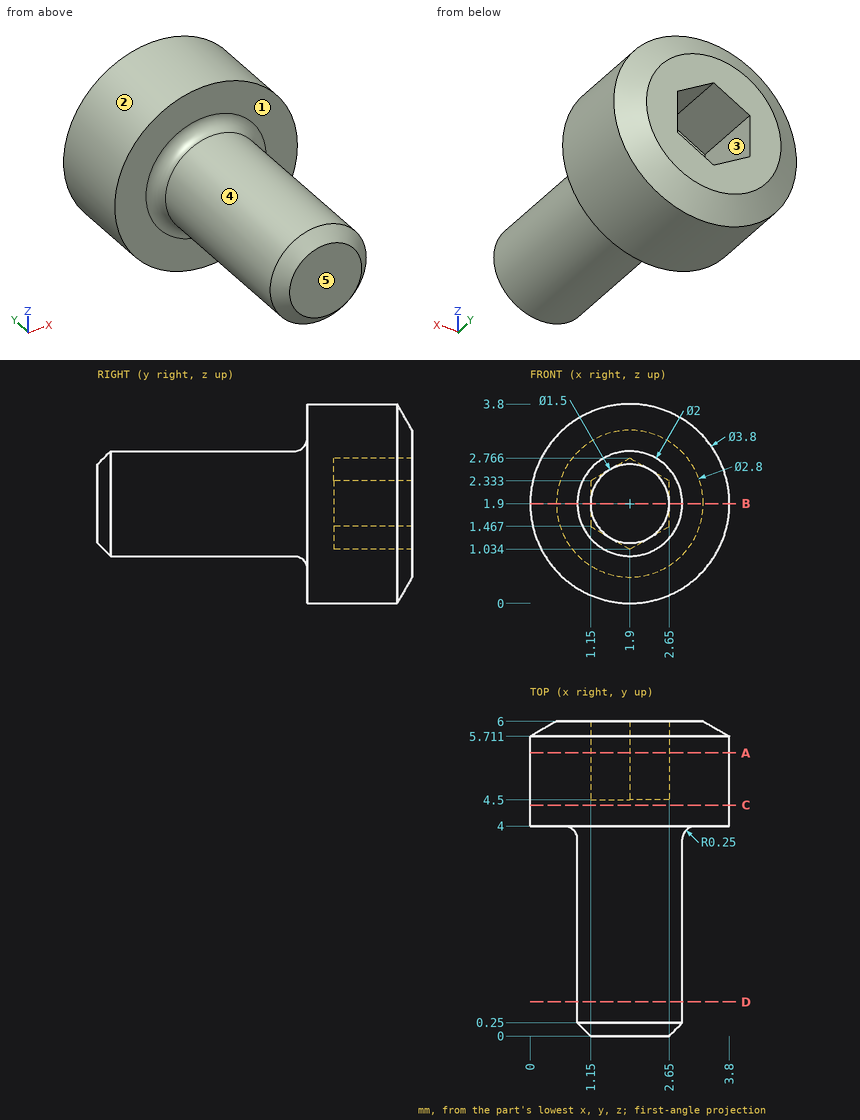
For this review, use the dimensioned drawing (mm, ordinates from the lowest corner) and the shaded views. A direction names the side the tool comes from. Give positions to 0.01 mm unless a question says otherwise; leave off trailing zeros. Order: outer loops, then holes, each group sorted by start corner. A loop starts at its lowest first (then second) coordinate and runs counter-clockwise, first axis right, second up.
1. Mouldability with a two-part tool opening along X and no side actions: class the marked faces 1, 2 and 3 as +X half, -X half, draft (parallel to the pull), parting line (faces both ways), or undercut.
Solution:
face 1: draft
face 2: parting line
face 3: undercut
2. Tool access review of the marked faces 4 and 5: name each direction out of +Z, -Z, +X, -X, +Y, -Y from which nothing blocks a thin tool from reaching the whole face with its end or side.
Solution:
face 4: -Y
face 5: +Z, -Z, +X, -X, -Y
3. Add section A-A, the plane y = 5.4. State the section outline as (x, z) points.
Solution:
outline: circle Ø3.8 at (1.9, 1.9); hole (1.15, 1.47) - (1.9, 1.03) - (2.65, 1.47) - (2.65, 2.33) - (1.9, 2.77) - (1.15, 2.33) - close
4. Add section C-C, the plane y = 4.4. State the section outline as (x, z) points.
Solution:
outline: circle Ø3.8 at (1.9, 1.9)
5. To check wall thickness, follow L1, parallel to Y at x = 3.2, z = 2.3; L2, parallel to Y at x = 2.05, z = 1.95; L3, parallel to Z at x = 1.95, y = 2.45. State the ranges of each line that lie inside material, in increasing order.
Solution:
L1: y = 4 to 6
L2: y = 0 to 4.5
L3: z = 0.9 to 2.9
6. Add section D-D, the plane y = 0.65. State the section outline as (x, z) points.
Solution:
outline: circle Ø2 at (1.9, 1.9)
7. Add section B-B, the plane z = 1.9. State the section outline as (x, y) points.
Solution:
outline: (0, 4) - (0.65, 4) arc R0.25 cw to (0.9, 3.75) - (0.9, 0.25) - (1.15, 0) - (2.65, 0) - (2.9, 0.25) - (2.9, 3.75) arc R0.25 cw to (3.15, 4) - (3.8, 4) - (3.8, 5.71) - (3.3, 6) - (2.65, 6) - (2.65, 4.5) - (1.15, 4.5) - (1.15, 6) - (0.5, 6) - (0, 5.71) - close
